```python
from build123d import *

# Parameters (mm, degrees)
SKETCH1_W                                       = 22.86
SKETCH1_H                                       = 15.24
BOSS_EXTRUDE1_DEPTH                             = 19.05
BOSS_EXTRUDE3_DEPTH                             = 3.81
LPATTERN1_COUNT                                 = 2
LPATTERN1_PITCH                                 = 11.43
SKETCH5_R                                       = 1.905
CUT_EXTRUDE2_DEPTH                              = 16.24
CUT_EXTRUDE3_DEPTH                              = 3.81
BOSS_EXTRUDE6_DEPTH                             = 3.175
SKETCH9_R                                       = 1.905
CUT_EXTRUDE4_DEPTH                              = 6.35
CUT_EXTRUDE5_DEPTH                              = 4.445
LPATTERN2_COUNT                                 = 2
LPATTERN2_PITCH                                 = 10.795
CBORE_FOR_6_PAN_HEAD_MACHINE_SCREW3_D           = 3.7500052
CBORE_FOR_6_PAN_HEAD_MACHINE_SCREW3_CBORE_D     = 7.5000104
CBORE_FOR_6_PAN_HEAD_MACHINE_SCREW3_CBORE_DEPTH = 2.032
SKETCH18_R                                      = 2.54
CUT_EXTRUDE8_DEPTH                              = 1.778
FILLET2_R                                       = 0.5
FILLET3_R                                       = 0.5
SKETCH19_W                                      = 3.111810153
SKETCH19_H                                      = 4.445
CUT_EXTRUDE9_DEPTH                              = 19.05
LPATTERN3_COUNT                                 = 2
LPATTERN3_PITCH                                 = 10.795
FILLET4_R                                       = 1


with BuildPart() as part:
    # Sketch1 → Boss-Extrude1 (new body)
    with BuildSketch(Plane(origin=(0, 0, 0), x_dir=(1, 0, 0), z_dir=(0, 1, 0))):
        Rectangle(SKETCH1_W, SKETCH1_H)
    extrude(amount=BOSS_EXTRUDE1_DEPTH)

    # Sketch3 → Boss-Extrude3 (add)
    with BuildSketch(Plane.XY.offset(7.62)):
        with BuildLine():
            Line((-11.43, 19.05), (-11.43, 0))
            ThreePointArc((-11.43, 0), (-19.521397873, 9.525), (-11.43, 19.05))
        make_face()
    boss_extrude3 = extrude(amount=-BOSS_EXTRUDE3_DEPTH)

    # LPattern1: Boss-Extrude3 ×2
    with Locations(*[(0, 0, -i * LPATTERN1_PITCH) for i in range(1, LPATTERN1_COUNT)]):
        add(boss_extrude3)

    # Sketch5 → Cut-Extrude2 (cut, through all)
    with BuildSketch(Plane.XY.offset(7.62)):
        with Locations((-9.869397873, 9.525)):
            Circle(SKETCH5_R)
    extrude(amount=-CUT_EXTRUDE2_DEPTH, mode=Mode.SUBTRACT)

    # Sketch6 → Cut-Extrude3 (cut, symmetric)
    with BuildSketch(Plane.XY):
        with BuildLine():
            Line((-11.43, 19.05), (-11.43, 0))
            ThreePointArc((-11.43, 0), (-0.217397873, 9.525), (-11.43, 19.05))
        make_face()
    extrude(amount=CUT_EXTRUDE3_DEPTH, both=True, mode=Mode.SUBTRACT)

    # Sketch8 → Boss-Extrude6 (add, symmetric)
    with BuildSketch(Plane.XY):
        with BuildLine():
            Line((11.43, 19.05), (11.43, 0))
            ThreePointArc((11.43, 0), (19.521397873, 9.525), (11.43, 19.05))
        make_face()
    extrude(amount=BOSS_EXTRUDE6_DEPTH, both=True)

    # Sketch9 → Cut-Extrude4 (cut)
    with BuildSketch(Plane.XY.offset(3.175)):
        with Locations(Location((11.901397873, 9.525, 0), (0, 0, 104.32684201))):  # turned: the seam where the file's is
            Circle(SKETCH9_R)
    extrude(amount=-CUT_EXTRUDE4_DEPTH, mode=Mode.SUBTRACT)

    # Sketch10 → Cut-Extrude5 (cut)
    with BuildSketch(Plane.XY.offset(3.175)):
        with BuildLine():
            Line((11.43, 19.05), (11.43, 0))
            ThreePointArc((11.43, 0), (0.217397873, 9.525), (11.43, 19.05))
        make_face()
    cut_extrude5 = extrude(amount=CUT_EXTRUDE5_DEPTH, mode=Mode.SUBTRACT)

    # LPattern2: Cut-Extrude5 ×2
    with Locations(*[(0, 0, -i * LPATTERN2_PITCH) for i in range(1, LPATTERN2_COUNT)]):
        add(cut_extrude5, mode=Mode.SUBTRACT)

    # CBORE for #6 Pan Head Machine Screw3 (through all)
    with Locations(Plane.XY.offset(7.62)):
        with Locations((-9.869397873, 9.525)):
            CounterBoreHole(CBORE_FOR_6_PAN_HEAD_MACHINE_SCREW3_D / 2, CBORE_FOR_6_PAN_HEAD_MACHINE_SCREW3_CBORE_D / 2, CBORE_FOR_6_PAN_HEAD_MACHINE_SCREW3_CBORE_DEPTH)

    # Sketch18 → Cut-Extrude8 (cut)
    with BuildSketch(Plane.XY.offset(5.588)):
        with Locations((-9.869397873, 9.525)):
            Circle(SKETCH18_R)
    extrude(amount=-CUT_EXTRUDE8_DEPTH, mode=Mode.SUBTRACT)

    # Fillet2
    fillet2_edges = [part.edges().sort_by_distance(p)[0] for p in [
        (-8.308795745, 19.05, 0),
        (-8.308795745, 0, 0),
    ]]
    fillet(fillet2_edges, radius=FILLET2_R)

    # Fillet3
    fillet3_edges = [part.edges().sort_by_distance(p)[0] for p in [
        (-13.619403073, 9.525, 7.62),
        (-13.619403073, 9.525, 5.588),
    ]]
    fillet(fillet3_edges, radius=FILLET3_R)

    # Sketch19 → Cut-Extrude9 (cut)
    with BuildSketch(Plane(origin=(0, 19.05, 0), x_dir=(1, 0, 0), z_dir=(0, 1, 0))):
        with Locations((6.752890669, -5.3975)):
            Rectangle(SKETCH19_W, SKETCH19_H)
    cut_extrude9 = extrude(amount=-CUT_EXTRUDE9_DEPTH, mode=Mode.SUBTRACT)

    # LPattern3: Cut-Extrude9 ×2
    with Locations(*[(0, 0, -i * LPATTERN3_PITCH) for i in range(1, LPATTERN3_COUNT)]):
        add(cut_extrude9, mode=Mode.SUBTRACT)

    # Fillet4
    fillet4_edges = [part.edges().sort_by_distance(p)[0] for p in [
        (5.196985592, 19.05, 5.3975),
        (5.196985592, 0, 5.3975),
        (5.196985592, 19.05, -5.3975),
        (5.196985592, 0, -5.3975),
    ]]
    fillet(fillet4_edges, radius=FILLET4_R)


solid = part.part
```
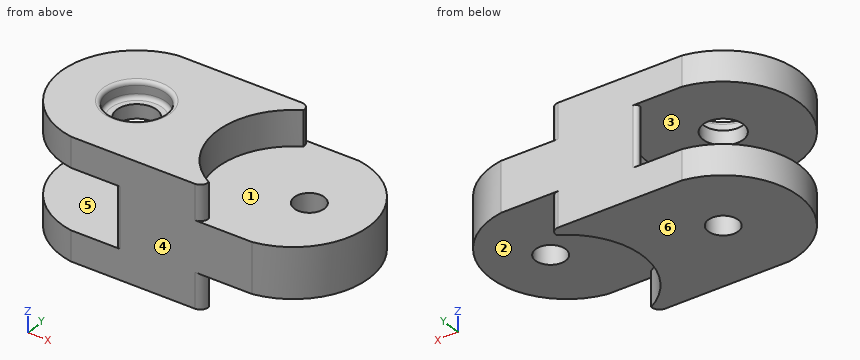
The model under review builds one solid part; all positions refer to its coordinate system, in mm. Face numbers are marked on the shaded views. A direction names the side the tool comes from. Round coordinates to 2 decimals unless told otherwise and drop trailing zeros. Loops run counter-clockwise (first coordinate to the right, second up) from the corner with the lowest first, then second, coordinate; pieces in that order, holes last. Notation, with made-up numbers: M -27,19.25 L -14,19.25 A31 cw -14,46.25 Z; hole C 2.25,67 d5. An arc over 180 degrees is marked long. Put each result on its own line as item: value.
Q1. Consider section B-B, the plane x = -15. Give the boundary of the cut face in (y, z).
Result set:
outline: M 1.35,-7.62 L 17.7,-7.62 L 17.7,-3.81 L 1.35,-3.81 Z; M 1.35,3.81 L 17.7,3.81 L 17.7,7.62 L 1.35,7.62 Z
Q2. Consider section A-A, the plane z = -5.5. Give the boundary of the cut face in (x, y) (3 decimals).
Result set:
outline: M -11.43,0 L 4.197,0 A1 ccw 5.197,1 L 5.197,1.079 A9.652 cw 5.197,17.971 L 5.197,18.05 A1 ccw 4.197,19.05 L -11.43,19.05 A9.652 ccw Z; hole C -9.869,9.525 d3.81
Q3. For pin 1 (8 mm diameter, centred on y = 2, z = -4, fed in from -X); pin 2 (9.5 mm diameter, centred on x = 6.5, y = 11.5, fed in from +Z) (3 decimals); pin 3 (2 mm diameter, centred on x = 7.5, y = 11, fed in from -Z) (3 decimals), all flat-tipped, find the tip position at first contact; note any pin that passes through.
Result set:
pin 1: stops at x = -18.85
pin 2: stops at z = 3.175
pin 3: stops at z = -3.175
Q4. Mouldability with a two-part tool opening along Z and no side actions: class the marked faces 4, 5 and 6 as released by +Z, released by -Z, zero draft, split by the parting line, or undercut.
Result set:
face 4: zero draft
face 5: undercut
face 6: released by -Z
Q5. Consider section C-C, the plane y = 1.5. Give the boundary of the cut face in (x, z) (3 decimals).
Result set:
outline: M -15.232,-7.62 L 4.507,-7.62 L 4.507,-3.175 L 15.232,-3.175 L 15.232,3.175 L 4.507,3.175 L 4.507,7.62 L -15.232,7.62 L -15.232,3.81 L -4.507,3.81 L -4.507,-3.81 L -15.232,-3.81 Z
Q6. To check wall thickness, follow L1, parallel to Z at x = -16, y = 3; L2, parallel to Z at x = 16, y = 13.5 (3 decimals); L3, parallel to Z at x = -8, y = 13. State the ranges of each line that lie inside material, in increasing order.
Result set:
L1: z = -7.62 to -3.81, 3.81 to 7.62
L2: z = -3.175 to 3.175
L3: z = -7.62 to -3.81, 3.81 to 7.52
Q7. Machinability: for the marked faces 1, 2 and 3, which of the approach directions +Z, -Z, +X, -X, +Y, -Y give a long, thin tool a straight path to every point of the face, cutting with its end or side? Answer none if there is none.
Result set:
face 1: +Z, +X
face 2: -Z, +X
face 3: -X
Q8. Consider section D-D, the plane x = -2.5. Give the boundary of the cut face in (y, z).
Result set:
outline: M 0,-7.62 L 19.05,-7.62 L 19.05,7.62 L 0,7.62 Z; hole M 3.29,-3.81 L 15.76,-3.81 L 15.76,3.81 L 3.29,3.81 Z
